Input: dimensioned drawing with shaded views. Units: mm. Origin: part minimum x, y, z. Give positions to 0.01 mm unless a question says otherwise; leave off trailing zeros. Order: outer loops, then holes, each group sorted by start corner. A loop starts at its lowest first (then second) coordinate and runs counter-clockwise, first axis right, second up.
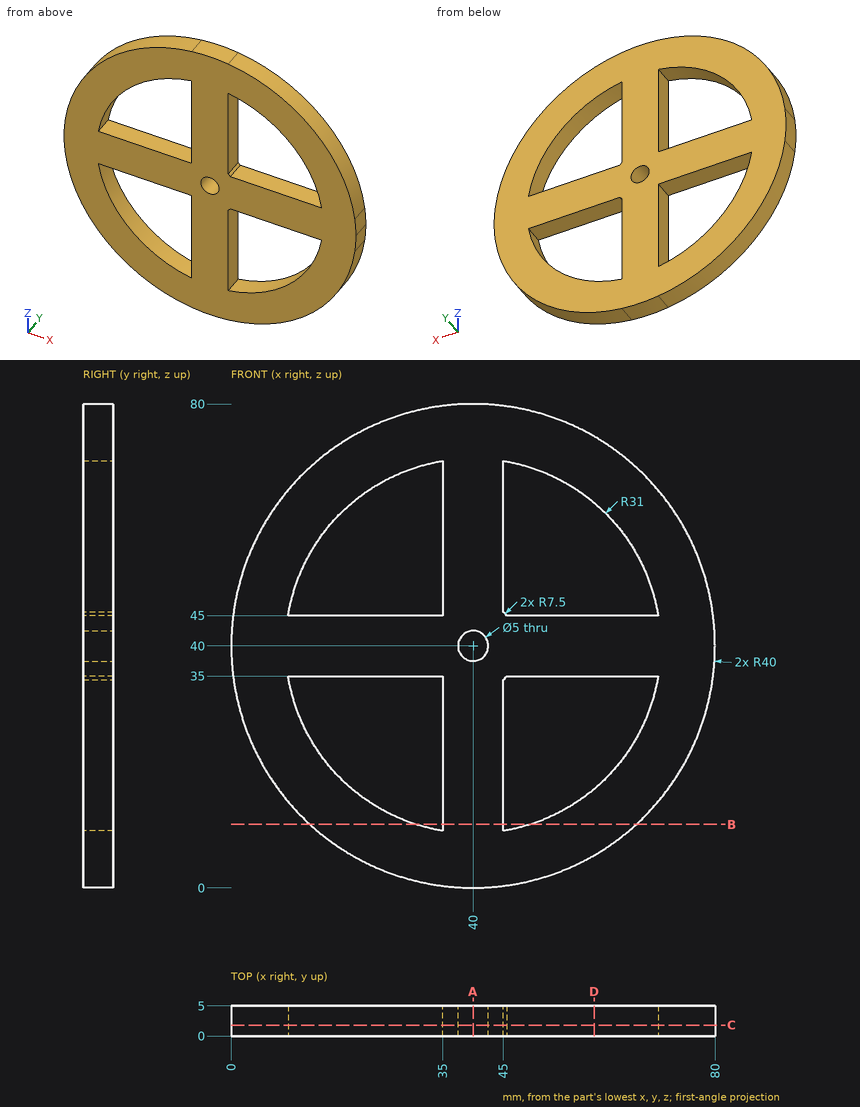
1) Material intervals for L1, parallel to X at y = 2.95, z = 61 (1 decimal); L2, parallel to Z at x = 28.5, y = 3.75; L3, parallel to X at y = 0.85, z = 64.5 (1 decimal), sorted ascending.
Report:
L1: x = 6 to 17.2, 35 to 45, 62.8 to 74
L2: z = 1.69 to 11.21, 35 to 45, 68.79 to 78.31
L3: x = 8.4 to 21, 35 to 45, 59 to 71.6
2) Pin query (flat end, axial travel): pin 1 (4 mm diameter, centred on x = 40, z = 40, fed in from -Y); pin 2 (2 mm diameter, centred on x = 12.5, y = 3.5, fed in from -Z); pin 3 (1.5 mm diameter, centred on y = 3.5, z = 51.5, fed in from -X); pin 4 (2.5 mm diameter, centred on x = 17.5, y = 3, fed in from +Z). Return the tip coordinate at first contact, or that it passes through.
Report:
pin 1: passes through
pin 2: stops at z = 10.04
pin 3: stops at x = 1.47
pin 4: stops at z = 73.89
3) Section query B-B, the plane z = 10.5. Return the cut outline in (x, y).
Report:
outline: (12.99, 0) - (30.47, 0) - (30.47, 5) - (12.99, 5) - close; (35, 0) - (45, 0) - (45, 5) - (35, 5) - close; (49.53, 0) - (67.01, 0) - (67.01, 5) - (49.53, 5) - close
4) Section query A-A, the plane x = 40. Return the cut outline in (y, z).
Report:
outline: (0, 0) - (5, 0) - (5, 37.5) - (0, 37.5) - close; (0, 42.5) - (5, 42.5) - (5, 80) - (0, 80) - close
5) Section query D-D, the plane x = 60. Return the cut outline in (y, z) (1 decimal).
Report:
outline: (0, 5.4) - (5, 5.4) - (5, 16.3) - (0, 16.3) - close; (0, 35) - (5, 35) - (5, 45) - (0, 45) - close; (0, 63.7) - (5, 63.7) - (5, 74.6) - (0, 74.6) - close
6) Section query C-C, the plane y = 1.8. Return the cut outline in (x, z).
Report:
outline: (0.31, 35) arc R40 ccw to (35, 0.31) arc R40 ccw to (45, 0.31) arc R40 ccw to (79.69, 35) arc R40 ccw to (80, 40) arc R40 ccw to (79.69, 45) arc R40 ccw to (45, 79.69) arc R40 ccw to (35, 79.69) arc R40 ccw to (0.31, 45) arc R40 ccw to start; hole (9.41, 35) arc R31 ccw to (35, 9.41) - (35, 35) - close; hole (9.41, 45) - (35, 45) - (35, 70.59) arc R31 ccw to start; hole circle Ø5 at (40, 40); hole (45, 9.41) arc R31 ccw to (70.59, 35) - (45.59, 35) arc R7.5 cw to (45, 34.41) - close; hole (45, 45.59) arc R7.5 cw to (45.59, 45) - (70.59, 45) arc R31 ccw to (45, 70.59) - close
